Part model, mm, in its own coordinate system. Face numbers are marked on the shaded views. A direction names the side the tool comes from. Coordinates: 2 decimals unless noted, no trailing zeros. Loops run counter-clockwise (first coordinate to the right, second up) from the corner with the lowest first, then second, coordinate; pieces in that order, holes last. Notation, with made-up numbers: M -7.5,-26.75 L 18.5,-26.75 A16 ccw 18.5,-5.75 Z; hole C 53.5,9.5 d10. An arc over 180 degrees is marked long. Answer as a JSON object with one key per item and string values. Group by question number.
1. Drill centre lines: L1, parallel to Z at x = -2, y = 7; L2, parallel to Y at x = 84, z = 36.5; L3, parallel to X at y = 17, z = 12. Where is each one in solid material? Low to high.
2. 3-axis set-ups, long thin cutter, end or side, ignore diameter. For the marked faces 4, 5, 6 and 7: which of +Z, -Z, +X, -X, +Y, -Y reach the whole face in a straight line?
3. Saw through at B-B on x = 76. Write the cut outline in (y, z), then the cut area to 3 significant figures.
4. Drop flat-ended pins along their axis: pin 1 Ø12.5 at (x, z) = (-10, 93.5) entering from -Y; pin 2 Ø6.5 at (y, z) = (43.5, 5) entering from -X; pin 3 Ø10 at (x, y) = (-72, 53.5) entering from +Z; pin 4 Ø10 at (y, z) = (62.5, 6.5) entering from +X. Give the stop position or say it passes through.
5. Saw through at C-C on z = 37. Write the cut outline in (x, y), then the cut area to 3 significant figures.
6. Saw through at D-D on y = 69.5. Write the cut outline in (x, z), then the cut area to 3 significant figures.
7. Saw through at A-A on y = 15.5. Write the cut outline in (x, z).
8. Mould opens along X. For the marked faces 1, 2 and 3 say: released by +X, released by -X, zero draft, split by the parting line, or undercut.
from build123d import *

# Parameters (mm, degrees)
F1_DEPTH = 101.6
F2_W     = 38.1
F2_H     = 31.75
F3_DEPTH = 25.4
F5_DEPTH = 76.2
F7_DEPTH = 50.8
F9_DEPTH = 127


with BuildPart() as f1:
    # F0 (on Front) → F1 (new body)
    with BuildSketch(Plane.XZ):
        with BuildLine():
            Line((-63.5, 0), (-38.1, 0))
            Line((-38.1, 0), (-38.1, 12.7))
            ThreePointArc((-38.1, 12.7), (-34.380256, 21.680256), (-25.4, 25.4))
            Line((-25.4, 25.4), (0, 25.4))
            Line((0, 25.4), (25.4, 25.4))
            ThreePointArc((25.4, 25.4), (34.380256, 21.680256), (38.1, 12.7))
            Line((38.1, 12.7), (38.1, 0))
            Line((38.1, 0), (63.5, 0))
            Line((63.5, 0), (63.5, 25.4))
            Line((63.5, 25.4), (101.6, 25.4))
            Line((101.6, 25.4), (101.6, 50.8))
            Line((101.6, 50.8), (0, 50.8))
            Line((0, 50.8), (-101.6, 50.8))
            Line((-101.6, 50.8), (-101.6, 25.4))
            Line((-101.6, 25.4), (-63.5, 25.4))
            Line((-63.5, 25.4), (-63.5, 0))
        make_face()
    extrude(amount=-F1_DEPTH)

    # F2 (on face) → F3 (cut)
    with BuildSketch(Plane.XY.offset(50.8)):
        with Locations((82.55, 47.625)):
            Rectangle(F2_W, F2_H)
        with Locations((-82.55, 47.625)):
            Rectangle(F2_W, F2_H)
    extrude(amount=-F3_DEPTH, mode=Mode.SUBTRACT)

    # F4 (on face) → F5 (join)
    with BuildSketch(Plane.XY.offset(50.8)):
        Polygon((50.8, 101.6), (-50.8, 101.6), (0, 0), align=None)
    extrude(amount=F5_DEPTH)

    # F6 (on Front) → F7 (cut)
    with BuildSketch(Plane.XZ):
        Polygon((-50.8, 76.2), (0, 76.2), (50.8, 76.2), (50.8, 101.6), (-50.8, 101.6), align=None)
    extrude(amount=-F7_DEPTH, mode=Mode.SUBTRACT)

    # F8 (on Top) → F9 (intersect, symmetric)
    with BuildSketch(Plane.XY):
        with BuildLine():
            Line((0, 101.6), (-88.9, 101.6))
            ThreePointArc((-88.9, 101.6), (-97.880256, 97.880256), (-101.6, 88.9))
            Line((-101.6, 88.9), (-101.6, 12.7))
            ThreePointArc((-101.6, 12.7), (-97.880256, 3.719744), (-88.9, 0))
            Line((-88.9, 0), (0, 0))
            Line((0, 0), (0, 101.6))
        make_face()
        with BuildLine():
            Line((88.9, 101.6), (0, 101.6))
            Line((0, 101.6), (0, 0))
            Line((0, 0), (88.9, 0))
            ThreePointArc((88.9, 0), (97.880256, 3.719744), (101.6, 12.7))
            Line((101.6, 12.7), (101.6, 88.9))
            ThreePointArc((101.6, 88.9), (97.880256, 97.880256), (88.9, 101.6))
        make_face()
    extrude(amount=F9_DEPTH, both=True, mode=Mode.INTERSECT)


solid = f1.part
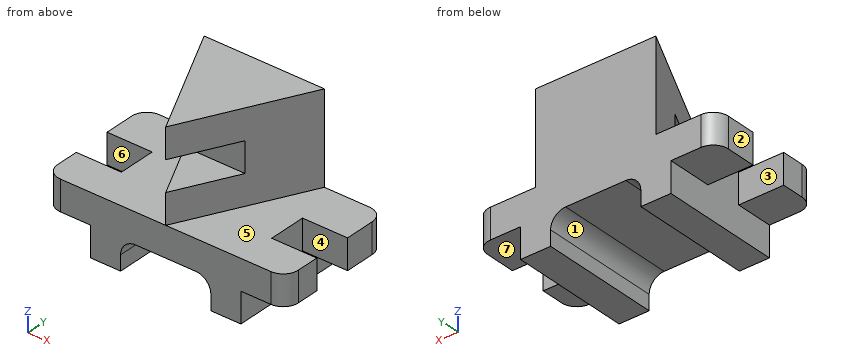
Outcome:
{
 "1": {"L1": "z = 25.4 to 76.2, 101.6 to 127", "L2": "y = 0 to 31.75, 63.5 to 101.6", "L3": "x = -63.5 to -38.1, 38.1 to 63.5"},
 "2": {"face 4": "+Z, -Z, +X", "face 5": "+Z, +X, -Y", "face 6": "+Z, -Z, -X", "face 7": "-Z, +X, +Y, -Y"},
 "3": {"outline": "M 0,25.4 L 31.75,25.4 L 31.75,50.8 L 0,50.8 Z; M 63.5,25.4 L 101.6,25.4 L 101.6,50.8 L 63.5,50.8 Z", "area": "1,770 mm²"},
 "4": {"pin 1": "stops at y = 50.8", "pin 2": "stops at x = -63.5", "pin 3": "passes through", "pin 4": "stops at x = 63.5"},
 "5": {"outline": "M -101.6,12.7 A12.7 ccw -88.9,0 L 88.9,0 A12.7 ccw 101.6,12.7 L 101.6,31.75 L 63.5,31.75 L 63.5,63.5 L 101.6,63.5 L 101.6,88.9 A12.7 ccw 88.9,101.6 L -88.9,101.6 A12.7 ccw -101.6,88.9 L -101.6,63.5 L -63.5,63.5 L -63.5,31.75 L -101.6,31.75 Z", "area": "18,100 mm²"},
 "6": {"outline": "M -101.6,25.4 L -63.5,25.4 L -63.5,0 L -38.1,0 L -38.1,12.7 A12.7 cw -25.4,25.4 L 25.4,25.4 A12.7 cw 38.1,12.7 L 38.1,0 L 63.5,0 L 63.5,25.4 L 101.6,25.4 L 101.6,50.8 L 34.75,50.8 L 34.75,127 L -34.75,127 L -34.75,50.8 L -101.6,50.8 Z", "area": "11,800 mm²"},
 "7": {"outline": "M -101.6,25.4 L -63.5,25.4 L -63.5,0 L -38.1,0 L -38.1,12.7 A12.7 cw -25.4,25.4 L 25.4,25.4 A12.7 cw 38.1,12.7 L 38.1,0 L 63.5,0 L 63.5,25.4 L 101.6,25.4 L 101.6,50.8 L 7.75,50.8 L 7.75,76.2 L -7.75,76.2 L -7.75,50.8 L -101.6,50.8 Z; M -7.75,101.6 L 7.75,101.6 L 7.75,127 L -7.75,127 Z"},
 "8": {"face 1": "undercut", "face 2": "released by -X", "face 3": "zero draft"}
}
